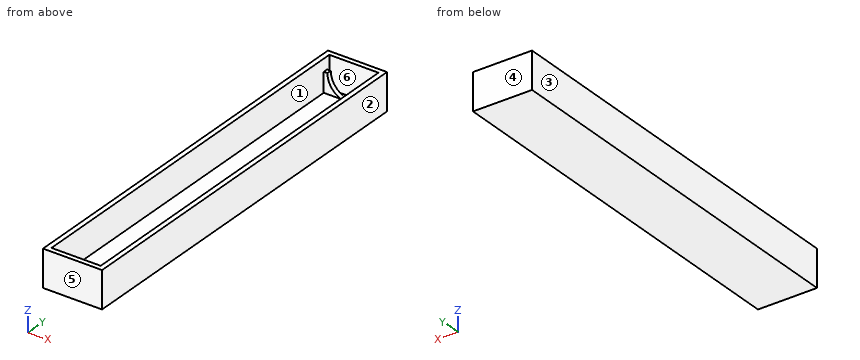
```python
from build123d import *

# Parameters (mm, degrees)
F0_W     = 24
F0_H     = 160
F1_DEPTH = 15
F2_T     = -2
F3_W     = 20
F3_H     = 1.90571
F4_DEPTH = 8
F5_R     = 8.5
F6_DEPTH = 2


with BuildPart() as f1:
    # F0 (on Top) → F1 (new body)
    with BuildSketch(Plane.XY):
        Rectangle(F0_W, F0_H)
    extrude(amount=F1_DEPTH)

    # F2
    f2_openings = [f1.faces().sort_by_distance(p)[0] for p in [
        (0, 0, 15),
    ]]
    offset(amount=F2_T, openings=f2_openings)

    # F3 (on face) → F4 (join)
    with BuildSketch(Plane.XY.offset(2)):
        with Locations((0, 75.811416)):
            Rectangle(F3_W, F3_H)
    extrude(amount=F4_DEPTH)

    # F5 (on face) → F6 (cut)
    with BuildSketch(Plane.XZ.offset(-74.858561)):
        with Locations((0, 10)):
            Circle(F5_R)
    extrude(amount=-F6_DEPTH, mode=Mode.SUBTRACT)


solid = f1.part
```
Design review of the part built by this model. Coordinates are the model's own, in mm. Face numbers are marked on the shaded views. A direction names the side the tool comes from. Coordinates: 2 decimals unless noted, no trailing zeros. Order: outer loops, then holes, each group sorted by start corner. A loop starts at its lowest first (then second) coordinate and runs counter-clockwise, first axis right, second up. Notation, with made-up numbers: M 63,87 L 86,87 A27 cw 86,114 Z; hole C 54,75 d8. An arc over 180 degrees is marked long. Answer as a JSON object with one key per item and string values. Group by question number.
1) Add section C-C, the plane x = 0. Write out the cut boundary in (y, z), then the cut area to 3 significant figures.
2) Mouldability with a two-part tool opening along X and no side actions: class the marked faces 1, 2, 3 and 4 as pulls with the +X half, pulls with the -X half, needs draft (parallel to the pull), parting line crosses it, or undercut.
3) Tool access review of the marked faces 5 and 6: name each direction out of +Z, -Z, +X, -X, +Y, -Y from which nothing blocks a thin tool from reaching the whole face with its end or side.
4) Add section D-D, the plane z = 13.25. Write out the cut boundary in (x, y), then the cut area to 3 significant figures.
5) Add section B-B, the plane y = -58.5. Write out the cut boundary in (x, z), then the cut area to 3 significant figures.
6) For pin 1 (1 mm diameter, centred on x = 3, y = 24, fed in from +Z), flat-tipped, find the tip position at first contact; note if it passes through.
7) Wall thickness on L1, parallel to Y at x = 8, z = 4; L2, parallel to X at y = -31.5, z = 2.75; L3, parallel to Y at x = 1, z = 14.25: over which ranges is each line inside the solid? List them lowest first.
8) Add section A-A, the plane z = 6. Write out the cut boundary in (x, y).
Computed values:
{
 "1": {"outline": "M -80,0 L 80,0 L 80,15 L 78,15 L 78,2 L 76.86,2 L 76.86,1.5 L 74.86,1.5 L 74.86,2 L -78,2 L -78,15 L -80,15 Z", "area": "371 mm^2"},
 "2": {"face 1": "undercut", "face 2": "pulls with the +X half", "face 3": "pulls with the -X half", "face 4": "needs draft"},
 "3": {"face 5": "+Z, -Z, +X, -X, -Y", "face 6": "+Z"},
 "4": {"outline": "M -12,-80 L 12,-80 L 12,80 L -12,80 Z; hole M -10,-78 L 10,-78 L 10,78 L -10,78 Z", "area": "720 mm^2"},
 "5": {"outline": "M -12,0 L 12,0 L 12,15 L 10,15 L 10,2 L -10,2 L -10,15 L -12,15 Z", "area": "100 mm^2"},
 "6": {"pin 1": "stops at z = 2"},
 "7": {"L1": "y = -80 to -78, 74.86 to 76.76, 78 to 80", "L2": "x = -12 to -10, 10 to 12", "L3": "y = -80 to -78, 78 to 80"},
 "8": {"outline": "M -12,-80 L 12,-80 L 12,80 L -12,80 Z; hole M -10,-78 L 10,-78 L 10,74.86 L 7.5,74.86 L 7.5,76.76 L 10,76.76 L 10,78 L -10,78 L -10,76.76 L -7.5,76.76 L -7.5,74.86 L -10,74.86 Z"}
}
